Source: CAD feature listing. Evaluate the final solid. Frame: model axes, mm. A direction names the side the tool comes from. Round coordinates to 2 decimals unless told otherwise and drop trailing zeros. Write each loop counter-clockwise with the first axis right and the second up, starting at its lowest first coordinate (ties: lowest second). Pieces come first, ordered by that corner, then holes. Notation, with made-up numbers: (25.25, -20) -> (80.25, -20) arc R35 ccw to (80.25, 15) -> close; hole circle Ø7 at (28.25, -31). An arc over 180 degrees is marked (long way). Put each result on its own line as item: value.
```python
from build123d import *

# Parameters (mm, degrees)
BOSS_EXTRU_1_DEPTH      = 1
ESQUISSE3_R             = 1.5
ENL_V_MAT_EXTRU_1_DEPTH = 1
ESQUISSE4_W             = 6
ESQUISSE4_H             = 4
BOSS_EXTRU_2_DEPTH      = 8.5
ESQUISSE7_W             = 10
ESQUISSE7_H             = 7.5
BOSS_EXTRU_4_DEPTH      = 5.5


with BuildPart() as part:
    # Esquisse1 → Boss.-Extru.1 (new body)
    with BuildSketch(Plane(origin=(0, 0, 0), x_dir=(1, 0, 0), z_dir=(0, 1, 0))):
        with BuildLine():
            Line((2, 0), (20, 0))
            ThreePointArc((20, 0), (21.414213562, 0.585786438), (22, 2))
            Line((22, 2), (22, 28))
            ThreePointArc((22, 28), (21.414213562, 29.414213562), (20, 30))
            Line((20, 30), (2, 30))
            ThreePointArc((2, 30), (0.585786438, 29.414213562), (0, 28))
            Line((0, 28), (0, 2))
            ThreePointArc((0, 2), (0.585786438, 0.585786438), (2, 0))
        make_face()
    extrude(amount=BOSS_EXTRU_1_DEPTH)

    # Esquisse3 → Enlèv. mat.-Extru.1 (cut)
    with BuildSketch(Plane(origin=(0, 1, 0), x_dir=(1, 0, 0), z_dir=(0, 1, 0))):
        with Locations((3, 27)):
            Circle(ESQUISSE3_R)
        with Locations((19, 27)):
            Circle(ESQUISSE3_R)
    extrude(amount=-ENL_V_MAT_EXTRU_1_DEPTH, mode=Mode.SUBTRACT)

    # Esquisse4 → Boss.-Extru.2 (add)
    with BuildSketch(Plane(origin=(0, 1, 0), x_dir=(1, 0, 0), z_dir=(0, 1, 0))):
        with Locations((11, 26.5)):
            Rectangle(ESQUISSE4_W, ESQUISSE4_H)
    extrude(amount=BOSS_EXTRU_2_DEPTH)

    # Esquisse6 → Révolution1 (revolve)
    with BuildSketch(Plane(origin=(11, 0, 0), x_dir=(0, 0, -1), z_dir=(1, 0, 0))):
        with BuildLine():
            Line((28.5, 6.5), (30, 6.5))
            ThreePointArc((30, 6.5), (29.596229956, 5.042262026), (28.5, 4))
            Line((28.5, 4), (28.5, 6.5))
        make_face()
    revolve(axis=Axis((11, 6.5, -28.5), (0, 0, -1)))

    # Esquisse7 → Boss.-Extru.4 (add)
    with BuildSketch(Plane(origin=(0, 1, 0), x_dir=(1, 0, 0), z_dir=(0, 1, 0))):
        with Locations((11, 4.25)):
            Rectangle(ESQUISSE7_W, ESQUISSE7_H)
    extrude(amount=BOSS_EXTRU_4_DEPTH)


solid = part.part
```
Q1. Cut plane B-B on x = 19. Output: boundary loops of the cut face in (y, z), and give its area (3 significant figures).
Ans:
outline: (0, -30) -> (1, -30) -> (1, -28.5) -> (0, -28.5) -> close; (0, -25.5) -> (1, -25.5) -> (1, 0) -> (0, 0) -> close
area: 27.0 mm^2
Q2. Cut plane A-A on y = 5. Output: boundary loops of the cut face in (x, z), and give its area (3 significant figures).
Ans:
outline: (6, -8) -> (16, -8) -> (16, -0.5) -> (6, -0.5) -> close; (8, -28.5) -> (9, -28.5) arc R2.4 ccw to (13, -28.5) -> (14, -28.5) -> (14, -24.5) -> (8, -24.5) -> close
area: 102 mm^2
Q3. Draft query along X for faces 1 (the cylindrical face through (17.89, 0.51, -28.01)), 2 (the flat face through (11, 0, -15)), 3 (the cylindrical face through (0.57, 0.49, -0.6)), 4 (the cylindrical face through (2.805, 0.507, -28.487)). Return one class per face: +X half, -X half, draft (parallel to the pull), parting line (faces both ways), or undercut.
Ans:
face 1: undercut
face 2: draft
face 3: -X half
face 4: undercut
Q4. Reachability of faces 5 (the flat face through (6, 4, -4)), 6 (the flat face through (11, 6.5, -4)), 7 (the flat face through (11, 5, -24.5)), 8 (the flat face through (16, 4, -4)) from +Z, -Z, +X, -X, +Y, -Y: full face, straight path, thin tool, end or side. Return the list, or none.
Ans:
face 5: +Z, -Z, -X, +Y
face 6: +Z, +X, -X, +Y
face 7: +X, -X, +Y
face 8: +Z, -Z, +X, +Y
Q5. Pin query (flat end, axial travel): pin 1 (3 mm diameter, centred on y = 6.5, z = -27, fed in from +X); pin 2 (3 mm diameter, centred on x = 15, z = -4, fed in from +Y); pin 3 (2 mm diameter, centred on y = 5.5, z = -26, fed in from -X); pin 4 (2.5 mm diameter, centred on x = 19, z = -27, fed in from +Y). Return the tip coordinate at first contact, or that it passes through.
Ans:
pin 1: stops at x = 14
pin 2: stops at y = 6.5
pin 3: stops at x = 8
pin 4: passes through
Q6. Cut plane D-D on z = -5.25. Output: boundary loops of the cut face in (x, y), and give its area (3 significant figures).
Ans:
outline: (0, 0) -> (22, 0) -> (22, 1) -> (16, 1) -> (16, 6.5) -> (6, 6.5) -> (6, 1) -> (0, 1) -> close
area: 77.0 mm^2
Q7. Cut plane C-C on z = -27. Output: boundary loops of the cut face in (x, y).
Ans:
outline: (0, 0) -> (1.5, 0) -> (1.5, 1) -> (0, 1) -> close; (4.5, 0) -> (17.5, 0) -> (17.5, 1) -> (14, 1) -> (14, 9.5) -> (8, 9.5) -> (8, 1) -> (4.5, 1) -> close; (20.5, 0) -> (22, 0) -> (22, 1) -> (20.5, 1) -> close
Q8. Material intervals for line 1 (X direction, y = 0.6, z = -27); line 2 (Z direction, x = 3, y = 0.75); line 3 (Z direction, x = 12.25, y = 3.75), sorted ascending. Write a range as [from, to].
Ans:
line 1: x = [0, 1.5], [4.5, 17.5], [20.5, 22]
line 2: z = [-30, -28.5], [-25.5, 0]
line 3: z = [-28.5, -24.5], [-8, -0.5]
